Check sheet for the drawn part. Datum: minimum x, y, z corner. Units: mm. A direction names the side the tool comes from. Round coordinates to 2 decimals unless told otherwise and drop trailing zeros. Write each loop counter-clockwise with the first axis right and the second up, starting at its lowest first coordinate (ties: lowest second). Pieces come first, ordered by that corner, then holes. Notation, with made-up numbers: (-13, 13.5) -> (19, 13.5) arc R25 cw to (19, 47.5) -> close; hole circle Ø1 at (-11, 76.5). An arc over 180 degrees is marked (long way). One line per item, written item: value. Start each with the question number.
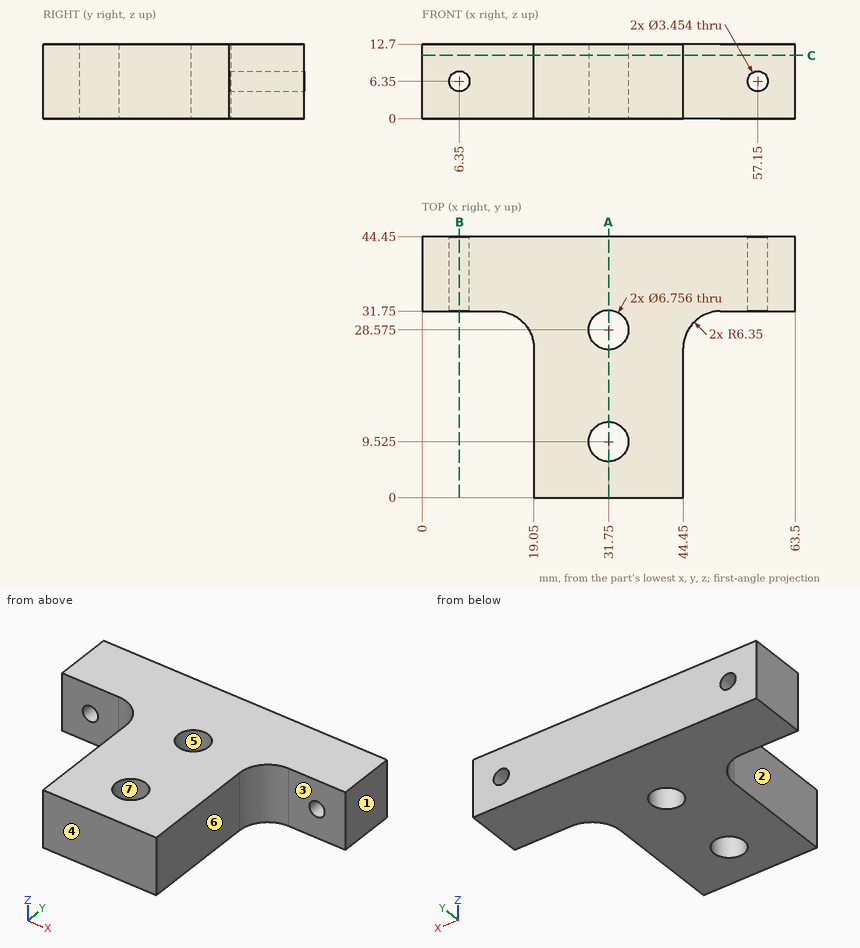
1. Cross-section at B-B (x = 6.35). Record the cut outline in (y, z).
2. Material ranges on probe 1 along Y at (x, z) = (31.75, 3.75); probe 2 along Z at (x, y) = (6.35, 35.5); probe 3 along X at (y, z) = (14, 1.5), recorded low to high.
3. Cross-section at C-C (z = 10.75). Give the number of separate pieces and of enclosed holes in the cut face, plus the area to 3 significant figures.
4. Cross-section at A-A (x = 31.75). Record the cut outline in (y, z).
5. Depth check by flat-ended pin: pin 1 Ø4 at (x, y) = (31.75, 28.575) entering from -Z; pin 2 Ø5.5 at (x, z) = (57.15, 6.35) entering from -Y; pin 3 Ø6.5 at (y, z) = (7, 6.5) entering from -X. Enter the tip coordinate at first touch or a pass-through.
6. Release check for a two-part mould opening along Y. For the marked faces 4, 5, 6 and 7 record: +Y half, -Y half, draft (parallel to the pull), parting line (faces both ways), or undercut.
7. Access from +Z, -Z, +X, -X, +Y, -Y to the whole of each face (thin tool, end or side, straight path). Record for the marked faces 1, 2 and 3.
Working result:
1. outline: (31.75, 0) -> (44.45, 0) -> (44.45, 4.62) -> (31.75, 4.62) -> close; (31.75, 8.08) -> (44.45, 8.08) -> (44.45, 12.7) -> (31.75, 12.7) -> close
2. probe 1: y = 0 to 6.15, 12.9 to 25.2, 31.95 to 44.45
2. probe 2: z = 0 to 4.62, 8.08 to 12.7
2. probe 3: x = 19.05 to 44.45
3. separate pieces: 1
3. enclosed holes: 2
3. area: 1,560 mm^2
4. outline: (0, 0) -> (6.15, 0) -> (6.15, 12.7) -> (0, 12.7) -> close; (12.9, 0) -> (25.2, 0) -> (25.2, 12.7) -> (12.9, 12.7) -> close; (31.95, 0) -> (44.45, 0) -> (44.45, 12.7) -> (31.95, 12.7) -> close
5. pin 1: passes through
5. pin 2: stops at y = 31.75
5. pin 3: stops at x = 19.05
6. face 4: -Y half
6. face 5: undercut
6. face 6: draft
6. face 7: undercut
7. face 1: +Z, -Z, +X, +Y, -Y
7. face 2: +Z, -Z, -X, -Y
7. face 3: +Z, -Z, +X, -Y
